The drawing under review shows one solid part. Ordinate dimensions are in mm from its lowest x, y, z. Coordinates: 2 decimals unless noted, no trailing zeros. Order: outer loops, then holes, each group sorted by start corner. A loop starts at its lowest first (then second) coordinate and runs counter-clockwise, first axis right, second up. Notation, with made-up numbers: (-14.5, 18.25) - (28.5, 18.25) arc R16 cw to (28.5, 34.25) - close; hole circle Ø8 at (-26, 77.25). An arc over 180 degrees is marked (long way). Answer in a Markdown table with one row per item.
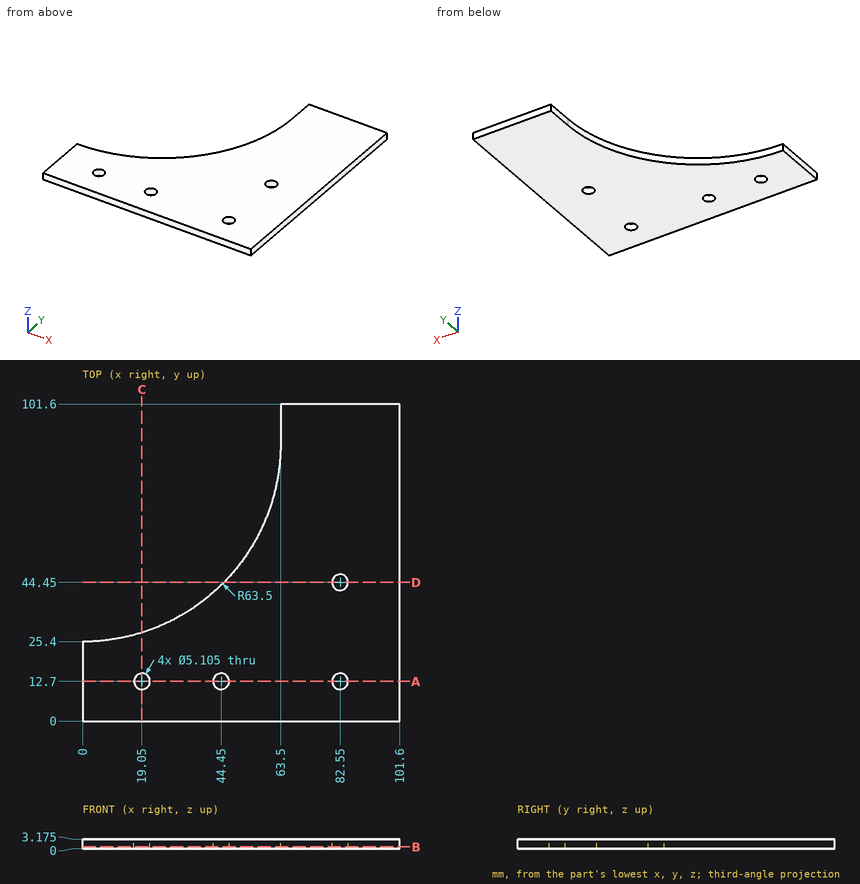
Item 1: We need section C-C, the plane x = 19.05. Write out the cut boundary in (y, z) (1 decimal).
Check values:
| item | result |
|---|---|
| outline | (0, 0) - (10.1, 0) - (10.1, 3.2) - (0, 3.2) - close; (15.3, 0) - (28.3, 0) - (28.3, 3.2) - (15.3, 3.2) - close |
Item 2: Clearance check with flat-ended pins moving along their axes: pin 1 Ø1 at (y, z) = (92.5, 2) entering from -X; pin 2 Ø1 at (y, z) = (36.5, 0.5) entering from -X (1 decimal). State where each tip first meets the part, or that it passes through.
Check values:
| item | result |
|---|---|
| pin 1 | x = 63.5 |
| pin 2 | x = 35.1 |
Item 3: We need section B-B, the plane z = 0.65. State how many separate pieces and enclosed holes the cut face has, then the cut area to 3 significant figures.
Check values:
| item | result |
|---|---|
| separate pieces | 1 |
| enclosed holes | 4 |
| area | 6,270 mm^2 |
Item 4: We need section D-D, the plane y = 44.45. Write out the cut boundary in (x, z) (1 decimal).
Check values:
| item | result |
|---|---|
| outline | (45.3, 0) - (80, 0) - (80, 3.2) - (45.3, 3.2) - close; (85.1, 0) - (101.6, 0) - (101.6, 3.2) - (85.1, 3.2) - close |
Item 5: To check wall thickness, follow line 1 (X direction, y = 12.7, z = 2.4); line 2 (X direction, y = 14.5, z = 1.95); line 3 (X direction, y = 95, z = 1.4). State the ranges of each line that lie inside material, in increasing order. Write a range as from..to.
Check values:
| item | result |
|---|---|
| line 1 | 0..16.5, 21.6..41.9, 47..80, 85.1..101.6 |
| line 2 | 0..17.24, 20.86..42.64, 46.26..80.74, 84.36..101.6 |
| line 3 | 63.5..101.6 |
Item 6: We need section A-A, the plane y = 12.7. Write out the cut boundary in (x, z) (1 decimal), then the cut area to 3 significant figures.
Check values:
| item | result |
|---|---|
| outline | (0, 0) - (16.5, 0) - (16.5, 3.2) - (0, 3.2) - close; (21.6, 0) - (41.9, 0) - (41.9, 3.2) - (21.6, 3.2) - close; (47, 0) - (80, 0) - (80, 3.2) - (47, 3.2) - close; (85.1, 0) - (101.6, 0) - (101.6, 3.2) - (85.1, 3.2) - close |
| area | 274 mm^2 |
